For this review, use the dimensioned drawing (mm, ordinates from the lowest corner) and the shaded views. A direction names the side the tool comes from. Coordinates: 2 decimals unless noted, no trailing zeros. Loops run counter-clockwise (first coordinate to the right, second up) from the corner with the lowest first, then second, coordinate; pieces in that order, holes last. Notation, with made-up numbers: M 54.25,88.5 L 76.25,88.5 A33 ccw 76.25,126.5 Z; hole C 40.5,-6.75 d1. An arc over 180 degrees is marked long. Write each question's results on one line, items separated by ' | '. Start each with the question number.
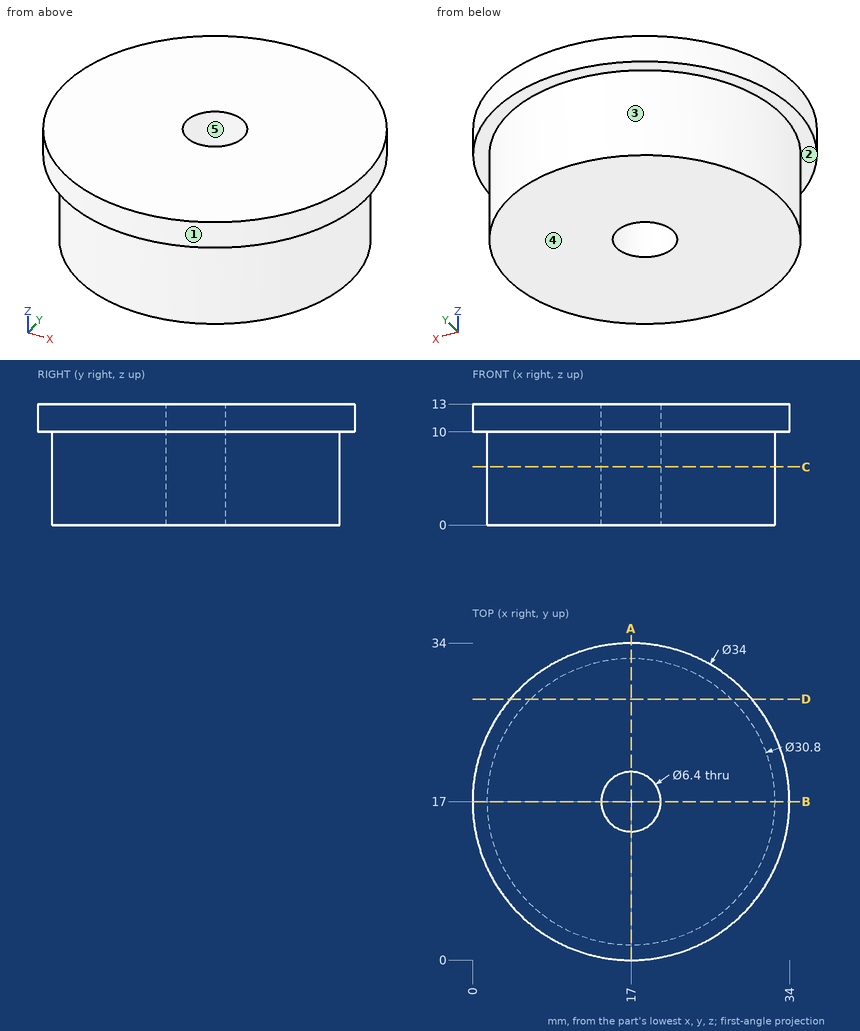
Q1. The part is to be moulded in two halves that separate along X. For the marked faces 3, 4 and 5, say which applies: pulls with the +X half, pulls with the -X half, needs draft (parallel to the pull), parting line crosses it, or undercut.
Q2. To check wall thickness, follow line 1 along Y through (x, z) = (17, 6.75); line 2 along Y through (x, z) = (19.5, 2); line 3 along X through (y, z) = (19, 6.5). State the ranges of each line that lie inside material, in increasing order.
Q3. For the marked faces 1 and 2, list the 3-axis set-ups (+Z, -Z, +X, -X, +Y, -Y) from which the entire face can be reached by the end or side of a thin tool; tool diameter is ignored.
Q4. Insertion check: P1, Ø1, axis at x = 26.5, z = 3, coming from the -Y side. The pin has a flat end and moves straight along its axis. Give the tip position at first contact, or say it passes through.
Q5. Take a section at C-C, the plane z = 6.25. Give the boundary of the cut face in (x, y).
Q6. Take a section at D-D, the plane y = 28. Give the boundary of the cut face in (x, z), then the cut area to 3 significant figures.
Q7. Take a section at A-A, the plane x = 17. Give the boundary of the cut face in (y, z), then the cut area to 3 significant figures.
Results:
1) face 3: parting line crosses it | face 4: needs draft | face 5: undercut
2) line 1: 1.6 to 13.8, 20.2 to 32.4 | line 2: 1.8 to 15, 19 to 32.2 | line 3: 1.73 to 14.5, 19.5 to 32.27
3) face 1: +Z, -Z | face 2: -Z
4) P1: y = 4.5
5) outline: C 17,17 d30.8; hole C 17,17 d6.4
6) outline: M 4.04,10 L 6.22,10 L 6.22,0 L 27.78,0 L 27.78,10 L 29.96,10 L 29.96,13 L 4.04,13 Z | area: 293 mm^2
7) outline: M 0,10 L 1.6,10 L 1.6,0 L 13.8,0 L 13.8,13 L 0,13 Z; M 20.2,0 L 32.4,0 L 32.4,10 L 34,10 L 34,13 L 20.2,13 Z | area: 327 mm^2
